from build123d import *

# Parameters (mm, degrees)
SKETCH_1_W      = 40
SKETCH_1_H      = 70
SKETCH_1_R      = 1.5
SKETCH_1_W_2    = 5
SKETCH_1_H_2    = 20
EXTRUDE_1_DEPTH = 10


with BuildPart() as part:
    # 草圖1 → 伸長1 (new body)
    with BuildSketch(Plane.XY):
        with Locations((0, 8.046617977)):
            Rectangle(SKETCH_1_W, SKETCH_1_H)
        with Locations((12.945335117, 29.143070151)):
            Circle(SKETCH_1_R, mode=Mode.SUBTRACT)
        with Locations((-12.945335117, 29.143070151)):
            Circle(SKETCH_1_R, mode=Mode.SUBTRACT)
        with Locations((0, -21.5)):
            Circle(SKETCH_1_R, mode=Mode.SUBTRACT)
        with Locations((0, 21.5)):
            Circle(SKETCH_1_R, mode=Mode.SUBTRACT)
        with Locations((12.5, 0)):
            Rectangle(SKETCH_1_W_2, SKETCH_1_H_2, mode=Mode.SUBTRACT)
    extrude(amount=EXTRUDE_1_DEPTH)


solid = part.part
Geometry: final body of the model. Coordinates: model frame, mm. A direction names the side the tool comes from. Give positions to 0.01 mm unless a question says otherwise; leave off trailing zeros. Order: outer loops, then holes, each group sorted by start corner. A loop starts at its lowest first (then second) coordinate and runs counter-clockwise, first axis right, second up. Notation, with made-up numbers: (-19.5, 61.25) -> (-5.5, 61.25) arc R24 cw to (-5.5, 76.25) -> close; hole circle Ø8 at (34, 54.5). An arc over 180 degrees is marked (long way). Answer as a JSON object with one key per item and string values.
Q1. Section C-C (z = 8.75). Output: boundary loops of the cut face in (x, y), plus the area to 3 significant figures.
Entries:
{"outline": "(-20, -26.95) -> (20, -26.95) -> (20, 43.05) -> (-20, 43.05) -> close; hole circle Ø3 at (-12.95, 29.14); hole circle Ø3 at (0, -21.5); hole circle Ø3 at (0, 21.5); hole (10, -10) -> (15, -10) -> (15, 10) -> (10, 10) -> close; hole circle Ø3 at (12.95, 29.14)", "area": "2,670 mm^2"}
Q2. Access query for faces 4 (the flat face through (12, 10, 5)), 5 (the flat face through (20, 8, 5)). Directions: +Z, -Z, +X, -X, +Y, -Y. A direction counts if a zero-diameter tool reaches every point of the face in a straight line with its end or side. Return the directions, or none.
Entries:
{"face 4": "+Z, -Z", "face 5": "+Z, -Z, +X, +Y, -Y"}
Q3. Material intervals for probe 1 along Y at (x, z) = (0, 6.25); probe 2 along Y at (x, z) = (10.5, 1.25); probe 3 along X at (y, z) = (-21, 8.5), sorted ascending.
Entries:
{"probe 1": "y = -26.95 to -23, -20 to 20, 23 to 43.05", "probe 2": "y = -26.95 to -10, 10 to 43.05", "probe 3": "x = -20 to -1.41, 1.41 to 20"}
Q4. Draft query along Y for faces 1 (the cylindrical face through (-13.27, 27.68, 4.93)), 2 (the flat face through (0, -26.953, 5)), 3 (the flat face through (-20, 8, 5)). Return one class per face: released by +Y, released by -Y, zero draft, split by the parting line, or undercut.
Entries:
{"face 1": "undercut", "face 2": "released by -Y", "face 3": "zero draft"}
Q5. Section B-B (y = 21.5). Output: boundary loops of the cut face in (x, z).
Entries:
{"outline": "(-20, 0) -> (-1.5, 0) -> (-1.5, 10) -> (-20, 10) -> close; (1.5, 0) -> (20, 0) -> (20, 10) -> (1.5, 10) -> close"}
Q6. Section A-A (x = 0). Output: boundary loops of the cut face in (y, z), plus the area to 3 significant figures.
Entries:
{"outline": "(-26.95, 0) -> (-23, 0) -> (-23, 10) -> (-26.95, 10) -> close; (-20, 0) -> (20, 0) -> (20, 10) -> (-20, 10) -> close; (23, 0) -> (43.05, 0) -> (43.05, 10) -> (23, 10) -> close", "area": "640 mm^2"}
